For this review, take the finished solid that the model builds, in its own axes (mm). Face numbers are marked on the shaded views. A direction names the side the tool comes from. Coordinates: 2 decimals unless noted, no trailing zeros. Write each loop counter-clockwise with the first axis right and the second up, starting at its lowest first coordinate (ties: lowest second). Pieces come first, ordered by that corner, then holes.
```python
from build123d import *

# Parameters (mm, degrees)
ESQUISSE1_R             = 10.16
ESQUISSE1_R_2           = 1.25
BOSS_EXTRU_2_DEPTH      = 3.81
BOSS_EXTRU_3_DEPTH      = 25.4
CHANFREIN1_SIZE         = 0.3175
ESQUISSE3_R             = 4.445
ENL_V_MAT_EXTRU_1_DEPTH = 2.54
ESQUISSE4_R             = 2.224538278
ENL_V_MAT_EXTRU_6_DEPTH = 2.794


with BuildPart() as part:
    # Esquisse1 → Boss.-Extru.2 (new body)
    with BuildSketch(Plane.XY):
        with Locations((0.618453307, -10.014969778)):
            Circle(ESQUISSE1_R)
        with Locations((8.589458927, -9.334477749)):
            Circle(ESQUISSE1_R_2, mode=Mode.SUBTRACT)
        with Locations((1.298945336, -17.985975399)):
            Circle(ESQUISSE1_R_2, mode=Mode.SUBTRACT)
        with Locations((-7.352552313, -10.695461808)):
            Circle(ESQUISSE1_R_2, mode=Mode.SUBTRACT)
        with Locations((-0.062038722, -2.043964158)):
            Circle(ESQUISSE1_R_2, mode=Mode.SUBTRACT)
    extrude(amount=BOSS_EXTRU_2_DEPTH)

    # Esquisse2 → Boss.-Extru.3 (add)
    with BuildSketch(Plane.XY.offset(3.81)):
        with BuildLine():
            Line((-1.286546693, -7.474969778), (2.523453307, -7.474969778))
            ThreePointArc((2.523453307, -7.474969778), (0.618453307, -13.189969778), (-1.286546693, -7.474969778))
        make_face()
    extrude(amount=BOSS_EXTRU_3_DEPTH)

    # Chanfrein1
    chanfrein1_edges = [part.edges().sort_by_distance(p)[0] for p in [
        (0.618453307, -13.189969778, 29.21),
        (-9.541546693, -10.014969778, 3.81),
    ]]
    chamfer(chanfrein1_edges, length=CHANFREIN1_SIZE)

    # Esquisse3 → Enlèv. mat.-Extru.1 (cut)
    with BuildSketch(Plane(origin=(0, 0, 0), x_dir=(-1, 0, 0), z_dir=(0, 0, -1))):
        with Locations((-0.618453307, -10.014969778)):
            Circle(ESQUISSE3_R)
    extrude(amount=-ENL_V_MAT_EXTRU_1_DEPTH, mode=Mode.SUBTRACT)

    # Esquisse4 → Enlèv. mat.-Extru.6 (cut)
    with BuildSketch(Plane.XY.offset(3.81)):
        with Locations((-0.062038722, -2.043964158)):
            Circle(ESQUISSE4_R)
        with Locations((8.589458927, -9.334477749)):
            Circle(ESQUISSE4_R)
        with Locations((1.298945336, -17.985975399)):
            Circle(ESQUISSE4_R)
        with Locations((-7.352552313, -10.695461808)):
            Circle(ESQUISSE4_R)
    extrude(amount=-ENL_V_MAT_EXTRU_6_DEPTH, mode=Mode.SUBTRACT)


solid = part.part
```
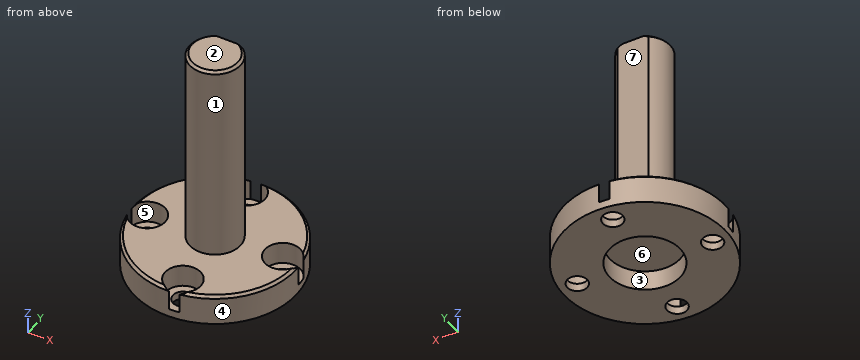
Q1. Add section B-B (z = 24). State the section outline as (x, y) points (3 decimals).
Ans:
outline: (-1.287, -7.475) arc R3.175 ccw (long way) to (2.523, -7.475) - close
Q2. Add section A-A (z = 2). State the section outline as (x, y) points (1 decimal).
Ans:
outline: (-9.5, -10.3) arc R2.2 cw (long way) to (-9.4, -11.5) arc R10.2 ccw to (0.9, -20.2) arc R2.2 cw (long way) to (2.1, -20.1) arc R10.2 ccw to (10.8, -9.7) arc R2.2 cw (long way) to (10.7, -8.6) arc R10.2 ccw to (0.4, 0.1) arc R2.2 cw (long way) to (-0.8, 0) arc R10.2 ccw to start; hole circle Ø8.9 at (0.6, -10)
Q3. Draft analysis for pull direction X (two halves, no side actions). For the marked faces 1, 2 and 3, state which applies: +X half, -X half, draft (parallel to the pull), parting line (faces both ways), or undercut.
Ans:
face 1: parting line
face 2: draft
face 3: undercut
Q4. For probe 1 along Z at (x, y) = (2.25, -4.5); probe 2 along Z at (x, y) = (-7.75, -9); probe 3 along Y at (x, z) = (-6, 2), list the stretches that pass through material, from the lowest coordinate up.
Ans:
probe 1: z = 0 to 3.81
probe 2: z = 0 to 1.02
probe 3: y = -17.72 to -12.46, -8.93 to -2.31
Q5. Clearance check with flat-ended pins moving along their axes: pin 1 Ø3.5 at (x, y) = (0.5, -2) entering from +Z; pin 2 Ø5 at (y, z) = (-14, 11) entering from -X; pin 3 Ø3 at (y, z) = (-14, 5.5) entering from -X. State where each tip first meets the part, or that it passes through.
Ans:
pin 1: stops at z = 3.81
pin 2: stops at x = -2.19
pin 3: stops at x = -1.36
Q6. Tool access review of the marked faces 4, 5, 6 and 7: name each direction out of +Z, -Z, +X, -X, +Y, -Y from which nothing blocks a thin tool from reaching the whole face with its end or side.
Ans:
face 4: +Z, -Z
face 5: +Z
face 6: -Z
face 7: +Z, +X, -X, +Y
